```python
from build123d import *

# Parameters (mm, degrees)
BOSS_EXTRU_1_DEPTH     = 120
SYM_TRIE6_COPY_1_DEPTH = 120


with BuildPart() as part:
    # Esquisse1 → Boss.-Extru.1 (new body)
    with BuildSketch(Plane.XY):
        with BuildLine():
            Line((-9.5, 10), (-4.58, 10))
            Line((-4.58, 10), (-3.125, 8.545))
            Line((-3.125, 8.545), (-3.125, 8.2))
            Line((-3.125, 8.2), (-5.5, 8.2))
            Line((-5.5, 8.2), (-5.5, 6.560660172))
            Line((-5.5, 6.560660172), (-2.839339828, 3.9))
            Line((-2.839339828, 3.9), (-0.21, 3.9))
            Line((-0.21, 3.9), (0, 3.69))
            Line((0, 3.69), (0, 2.1))
            ThreePointArc((0, 2.1), (-2.1, 0), (0, -2.1))
            Line((0, -2.1), (0, -3.69))
            Line((0, -3.69), (-0.21, -3.9))
            Line((-0.21, -3.9), (-2.839339828, -3.9))
            Line((-2.839339828, -3.9), (-6.239339828, -7.3))
            Line((-6.239339828, -7.3), (-8.2, -7.3))
            Line((-8.2, -7.3), (-8.2, -10))
            Line((-8.2, -10), (-10, -10))
            Line((-10, -10), (-10, -4.58))
            Line((-10, -4.58), (-8.545, -3.125))
            Line((-8.545, -3.125), (-8.2, -3.125))
            Line((-8.2, -3.125), (-8.2, -5.5))
            Line((-8.2, -5.5), (-6.560660172, -5.5))
            Line((-6.560660172, -5.5), (-3.9, -2.839339828))
            Line((-3.9, -2.839339828), (-3.9, -0.21))
            Line((-3.9, -0.21), (-3.69, 0))
            Line((-3.69, 0), (-3.9, 0.21))
            Line((-3.9, 0.21), (-3.9, 2.839339828))
            Line((-3.9, 2.839339828), (-6.560660172, 5.5))
            Line((-6.560660172, 5.5), (-8.2, 5.5))
            Line((-8.2, 5.5), (-8.2, 3.125))
            Line((-8.2, 3.125), (-8.545, 3.125))
            Line((-8.545, 3.125), (-10, 4.58))
            Line((-10, 4.58), (-10, 9.5))
            ThreePointArc((-10, 9.5), (-9.853553391, 9.853553391), (-9.5, 10))
        make_face()
    boss_extru_1 = extrude(amount=BOSS_EXTRU_1_DEPTH)

    # Sym_trie1: Boss.-Extru.1 across plane
    add(boss_extru_1.mirror(Plane(origin=(0, 3.69, 120), x_dir=(0, 0, 1), z_dir=(-1, 0, 0))))

    # Sym_trie6: Boss.-Extru.1 across plane
    add(boss_extru_1.mirror(Plane(origin=(-8.2, -10, 120), x_dir=(0, 0, 1), z_dir=(0, 1, 0))))

    # Sym_trie6 copy 1 sketch → Sym_trie6 copy 1 (add)
    with BuildSketch(Plane(origin=(0, -20, 0), x_dir=(-1, 0, 0), z_dir=(0, 0, 1))):
        with BuildLine():
            Line((-9.5, 10), (-4.58, 10))
            Line((-4.58, 10), (-3.125, 8.545))
            Line((-3.125, 8.545), (-3.125, 8.2))
            Line((-3.125, 8.2), (-5.5, 8.2))
            Line((-5.5, 8.2), (-5.5, 6.560660172))
            Line((-5.5, 6.560660172), (-2.839339828, 3.9))
            Line((-2.839339828, 3.9), (-0.21, 3.9))
            Line((-0.21, 3.9), (0, 3.69))
            Line((0, 3.69), (0, 2.1))
            ThreePointArc((0, 2.1), (-2.1, 0), (0, -2.1))
            Line((0, -2.1), (0, -3.69))
            Line((0, -3.69), (-0.21, -3.9))
            Line((-0.21, -3.9), (-2.839339828, -3.9))
            Line((-2.839339828, -3.9), (-6.239339828, -7.3))
            Line((-6.239339828, -7.3), (-8.2, -7.3))
            Line((-8.2, -7.3), (-8.2, -10))
            Line((-8.2, -10), (-10, -10))
            Line((-10, -10), (-10, -4.58))
            Line((-10, -4.58), (-8.545, -3.125))
            Line((-8.545, -3.125), (-8.2, -3.125))
            Line((-8.2, -3.125), (-8.2, -5.5))
            Line((-8.2, -5.5), (-6.560660172, -5.5))
            Line((-6.560660172, -5.5), (-3.9, -2.839339828))
            Line((-3.9, -2.839339828), (-3.9, -0.21))
            Line((-3.9, -0.21), (-3.69, 0))
            Line((-3.69, 0), (-3.9, 0.21))
            Line((-3.9, 0.21), (-3.9, 2.839339828))
            Line((-3.9, 2.839339828), (-6.560660172, 5.5))
            Line((-6.560660172, 5.5), (-8.2, 5.5))
            Line((-8.2, 5.5), (-8.2, 3.125))
            Line((-8.2, 3.125), (-8.545, 3.125))
            Line((-8.545, 3.125), (-10, 4.58))
            Line((-10, 4.58), (-10, 9.5))
            ThreePointArc((-10, 9.5), (-9.853553391, 9.853553391), (-9.5, 10))
        make_face()
    extrude(amount=SYM_TRIE6_COPY_1_DEPTH)


solid = part.part
```
The listing builds one solid part. Answer for the finished solid, in the listing's coordinates (mm). A direction names the side the tool comes from. Give positions to 0.01 mm unless a question says otherwise; leave off trailing zeros. Order: outer loops, then holes, each group sorted by start corner. A loop starts at its lowest first (then second) coordinate and runs counter-clockwise, first axis right, second up. Notation, with made-up numbers: (30, 50) -> (66, 50) arc R24 cw to (66, 68) -> close; hole circle Ø11 at (2, -23.75). An arc over 180 degrees is marked (long way). One line per item, written item: value.
1) Determine the mould class of faces 4 (the flat face through (-5, -15, 0)), 5 (the flat face through (10, 7, 59)), 6 (the flat face through (-4.52, -14.42, 59.16)) for opening direction X: pulls with the +X half, pulls with the -X half, needs draft (parallel to the pull), parting line crosses it, or undercut.
Reported:
face 4: needs draft
face 5: pulls with the +X half
face 6: undercut
2) Find the intervals of material crossed by line 1 (Y direction, x = 0, z = 58.5); line 2 (Y direction, x = -8.5, z = 6.5) (3 decimals); line 3 (X direction, y = -20, z = 65), in increasing order.
Reported:
line 1: y = -23.69 to -22.1, -17.9 to -16.31, -3.69 to -2.1, 2.1 to 3.69
line 2: y = -30 to -23.125, -16.875 to -3.125, 3.125 to 10
line 3: x = -3.69 to -2.1, 2.1 to 3.69
3) Find section A-A, the plane y = -10.5. Determine the outline of the cut face in (x, z).
Reported:
outline: (-10, 0) -> (-8.2, 0) -> (-8.2, 120) -> (-10, 120) -> close; (8.2, 0) -> (10, 0) -> (10, 120) -> (8.2, 120) -> close
4) Flat-ended cylindrical pins translate along their axes: P1, Ø1.5, axis at x = -3.5, z = 66.5, coming from the -Y side; P2, Ø0.8, axis at y = 2, z = 30, coming from the -X side; P3, Ø4, axis at y = -21.5, z = 18.5, coming from the -X side. Find the tip coordinate at first contact, or state that the pin passes through.
Reported:
P1: stops at y = -29.67
P2: stops at x = -3.9
P3: stops at x = -8.92
5) A tool of negligible diameter and unlimited length cuts with its end or side. For faces 1 (the flat face through (-10, -10, 59)), 2 (the flat face through (2, 3.9, 59)), 3 (the flat face through (-4.52, -5.58, 59.16)), from which of +Z, -Z, +X, -X, +Y, -Y can it reach the whole face along a straight path? Write none if from no direction.
Reported:
face 1: +Z, -Z, -X, +Y, -Y
face 2: +Z, -Z, +Y
face 3: +Z, -Z
6) Find section B-B, the plane z = 32. Count the separate pieces of the cut face and the enclosed holes in it, plus the area to 3 significant figures.
Reported:
separate pieces: 1
enclosed holes: 3
area: 300 mm^2
